Here's how the part is built. I have some questions about the finished solid (model axes, mm). A direction names the side the tool comes from. Round coordinates to 2 decimals unless told otherwise and drop trailing zeros. Order: outer loops, then holes, each group sorted by start corner. A loop starts at its lowest first (then second) coordinate and runs counter-clockwise, first axis right, second up.
```python
from build123d import *

# Parameters (mm, degrees)
BOSS_EXTRUDE1_DEPTH     = 3
BOSS_EXTRUDE2_DEPTH     = 132
CUT_EXTRUDE1_DEPTH      = 219.5
CUT_EXTRUDE1_DEPTH_BACK = 24.5
SKETCH3_W               = 129
SKETCH3_H               = 210
CUT_EXTRUDE2_DEPTH      = 322
CUT_EXTRUDE2_DEPTH_BACK = 22
SKETCH5_W               = 145
SKETCH5_H               = 129
BOSS_EXTRUDE3_DEPTH     = 10
BOSS_EXTRUDE4_DEPTH     = 15
CHAMFER1_SIZE           = 5
CHAMFER2_SIZE           = 3
CUT_EXTRUDE3_DEPTH      = 295
CUT_EXTRUDE3_DEPTH_BACK = 5
SKETCH10_R              = 2.5
SKETCH11_R              = 12
SKETCH11_R_2            = 7.6
SKETCH11_R_3            = 25
SKETCH11_R_4            = 1.6
CUT_EXTRUDE4_DEPTH      = 10
SKETCH13_R              = 4
CUT_EXTRUDE6_DEPTH      = 10


with BuildPart() as part:
    # Sketch1 → Boss-Extrude1 (new body)
    with BuildSketch(Plane.XY):
        with BuildLine():
            Line((15, 0), (235, 0))
            ThreePointArc((235, 0), (245.606601718, 4.393398282), (250, 15))
            Line((250, 15), (250, 335))
            ThreePointArc((250, 335), (245.606601718, 345.606601718), (235, 350))
            Line((235, 350), (15, 350))
            ThreePointArc((15, 350), (4.393398282, 345.606601718), (0, 335))
            Line((0, 335), (0, 15))
            ThreePointArc((0, 15), (4.393398282, 4.393398282), (15, 0))
        make_face()
    extrude(amount=BOSS_EXTRUDE1_DEPTH)

    # Sketch2 → Boss-Extrude2 (add)
    with BuildSketch(Plane.XY.offset(3)):
        with BuildLine():
            Line((0, 335), (0, 15))
            ThreePointArc((0, 15), (4.393398282, 4.393398282), (15, 0))
            Line((15, 0), (235, 0))
            ThreePointArc((235, 0), (245.606601718, 4.393398282), (250, 15))
            Line((250, 15), (250, 335))
            ThreePointArc((250, 335), (245.606601718, 345.606601718), (235, 350))
            Line((235, 350), (15, 350))
            ThreePointArc((15, 350), (4.393398282, 345.606601718), (0, 335))
        make_face()
        with BuildLine():
            ThreePointArc((32.5, 325), (28.964466094, 323.535533906), (27.5, 320))
            Line((27.5, 320), (27.5, 30))
            ThreePointArc((27.5, 30), (28.964466094, 26.464466094), (32.5, 25))
            Line((32.5, 25), (217.5, 25))
            ThreePointArc((217.5, 25), (221.035533906, 26.464466094), (222.5, 30))
            Line((222.5, 30), (222.5, 320))
            ThreePointArc((222.5, 320), (221.035533906, 323.535533906), (217.5, 325))
            Line((217.5, 325), (32.5, 325))
        make_face(mode=Mode.SUBTRACT)
    extrude(amount=BOSS_EXTRUDE2_DEPTH)

    # Sketch3 → Cut-Extrude1 (cut, two sides: drawn at the far end of the back side and taken through both)
    with BuildSketch(Plane(origin=(27.5, 0, 0), x_dir=(0, 0, -1), z_dir=(1, 0, 0)).offset(-CUT_EXTRUDE1_DEPTH_BACK)):
        with Locations((-67.5, 175)):
            Rectangle(SKETCH3_W, SKETCH3_H)
    extrude(amount=CUT_EXTRUDE1_DEPTH + CUT_EXTRUDE1_DEPTH_BACK, mode=Mode.SUBTRACT)

    # Sketch5 → Cut-Extrude2 (cut, two sides: drawn at the far end of the back side and taken through both)
    with BuildSketch(Plane(origin=(0, 25, 0), x_dir=(1, 0, 0), z_dir=(0, 1, 0)).offset(-CUT_EXTRUDE2_DEPTH_BACK)):
        with Locations((125, -67.5)):
            Rectangle(SKETCH5_W, SKETCH5_H)
    extrude(amount=CUT_EXTRUDE2_DEPTH + CUT_EXTRUDE2_DEPTH_BACK, mode=Mode.SUBTRACT)

    # Sketch8 → Boss-Extrude3 (add)
    with BuildSketch(Plane.XY.offset(135)):
        with BuildLine():
            Line((225.5, 30), (225.5, 320))
            ThreePointArc((225.5, 320), (223.156854249, 325.656854249), (217.5, 328))
            Line((217.5, 328), (32.5, 328))
            ThreePointArc((32.5, 328), (26.843145751, 325.656854249), (24.5, 320))
            Line((24.5, 320), (24.5, 30))
            ThreePointArc((24.5, 30), (26.843145751, 24.343145751), (32.5, 22))
            Line((32.5, 22), (217.5, 22))
            ThreePointArc((217.5, 22), (223.156854249, 24.343145751), (225.5, 30))
        make_face()
        with BuildLine():
            Line((32.5, 25), (217.5, 25))
            ThreePointArc((217.5, 25), (221.035533906, 26.464466094), (222.5, 30))
            Line((222.5, 30), (222.5, 320))
            ThreePointArc((222.5, 320), (221.035533906, 323.535533906), (217.5, 325))
            Line((217.5, 325), (32.5, 325))
            ThreePointArc((32.5, 325), (28.964466094, 323.535533906), (27.5, 320))
            Line((27.5, 320), (27.5, 30))
            ThreePointArc((27.5, 30), (28.964466094, 26.464466094), (32.5, 25))
        make_face(mode=Mode.SUBTRACT)
    extrude(amount=BOSS_EXTRUDE3_DEPTH)

    # Sketch9 → Boss-Extrude4 (add)
    with BuildSketch(Plane.XY.offset(135)):
        with BuildLine():
            ThreePointArc((0, 15), (4.393398282, 4.393398282), (15, 0))
            Line((15, 0), (30, 0))
            Line((30, 0), (30, 15))
            Line((30, 15), (15, 30))
            Line((15, 30), (0, 30))
            Line((0, 30), (0, 15))
        make_face()
        with BuildLine():
            Line((0, 335), (0, 320))
            Line((0, 320), (15, 320))
            Line((15, 320), (30, 335))
            Line((30, 335), (30, 350))
            Line((30, 350), (15, 350))
            ThreePointArc((15, 350), (4.393398282, 345.606601718), (0, 335))
        make_face()
    extrude(amount=BOSS_EXTRUDE4_DEPTH)

    # Chamfer1
    chamfer1_edges = [part.edges().sort_by_distance(p)[0] for p in [
        (0, 22.5, 150),
        (4.393398282, 4.393398282, 150),
        (22.5, 0, 150),
        (22.5, 350, 150),
        (4.393398282, 345.606601718, 150),
        (0, 327.5, 150),
    ]]
    chamfer(chamfer1_edges, length=CHAMFER1_SIZE)

    # Chamfer2
    chamfer2_edges = [part.edges().sort_by_distance(p)[0] for p in [
        (30, 10, 150),
        (22.5, 22.5, 150),
        (22.5, 327.5, 150),
        (30, 340, 150),
        (10, 30, 150),
        (10, 320, 150),
    ]]
    chamfer(chamfer2_edges, length=CHAMFER2_SIZE)

    # Sketch10 → Cut-Extrude3 (cut, two sides: drawn at the far end of the back side and taken through both)
    with BuildSketch(Plane(origin=(0, 30, 0), x_dir=(1, 0, 0), z_dir=(0, 1, 0)).offset(-CUT_EXTRUDE3_DEPTH_BACK)):
        with Locations(Location((7, -144, 0), (0, 0, 270))):
            Circle(SKETCH10_R)
    extrude(amount=CUT_EXTRUDE3_DEPTH + CUT_EXTRUDE3_DEPTH_BACK, mode=Mode.SUBTRACT)

    # Sketch11 → Cut-Extrude4 (cut)
    with BuildSketch(Plane(origin=(0, 3, 0), x_dir=(1, 0, 0), z_dir=(0, 1, 0))):
        with Locations(Location((160, -87.5, 0), (0, 0, 270))):
            Circle(SKETCH11_R)
        with Locations(Location((145, -47.5, 0), (0, 0, 270))):
            Circle(SKETCH11_R_2)
        with Locations(Location((175, -47.5, 0), (0, 0, 270))):
            Circle(SKETCH11_R_2)
        with Locations(Location((90, -67.5, 0), (0, 0, 270))):
            Circle(SKETCH11_R_3)
        with Locations(Location((150.5, -99.5, 0), (0, 0, 270))):
            Circle(SKETCH11_R_4)
        with Locations(Location((169.5, -75.5, 0), (0, 0, 270))):
            Circle(SKETCH11_R_4)
    extrude(amount=-CUT_EXTRUDE4_DEPTH, mode=Mode.SUBTRACT)

    # Sketch13 → Cut-Extrude6 (cut)
    with BuildSketch(Plane.ZY.offset(-247)):
        with Locations((67.5, 140)):
            Circle(SKETCH13_R)
        with BuildLine():
            Line((57.460079682, 173.9), (56.5, 173.9))
            Line((56.5, 173.9), (56.5, 176.1))
            Line((56.5, 176.1), (57.460079682, 176.1))
            ThreePointArc((57.460079682, 176.1), (77.6, 175), (57.460079682, 173.9))
        make_face()
    extrude(amount=-CUT_EXTRUDE6_DEPTH, mode=Mode.SUBTRACT)


solid = part.part
```
1. On a 3-axis mill with a long thin cutter (end or side, diameter ignored), from which of +Z, -Z, +X, -X, +Y, -Y can I reach the whole of each face in a straight line? I mean faces 1 (the cylindrical face through (248.48, 175.43, 77.59)), 2 (the flat face through (15, 174, 132)), 3 (the flat face through (234, 177, 135)), 4 (the flat face through (21.56, 21.35, 148.48)). Say none if no direction works.
Evaluation:
face 1: +X
face 2: none
face 3: +Z
face 4: +Z, +X
2. If we mould it in two halves opening along Y, with no side actions, what happens to faces 5 (the flat face through (197.5, 14, 68)), 6 (the flat face through (30, 7, 141)), 7 (the cylindrical face through (248.479, 143.373, 69.65)), 8 (the cylindrical face through (4.28, 4.51, 71.48))? For each: released by +Y, released by -Y, zero draft, split by the parting line, or undercut.
Evaluation:
face 5: undercut
face 6: zero draft
face 7: undercut
face 8: released by -Y
3. I'm going to push flat-ended pins straight in: P1, Ø3, axis at y = 120, z = 142.5, coming from the -X side; P2, Ø9.5, axis at y = 340.5, z = 143.5, coming from the +X side; P3, Ø10, axis at x = 98, y = 95.5, coming from the +Z side. Where does each tip first touch, or does it pass through?
Evaluation:
P1: stops at x = 24.5
P2: stops at x = 30
P3: stops at z = 3
4. If we section it at A-A, the plane x = 110: Write out the boundary of the cut face in (y, z).
Evaluation:
outline: (0, 0) - (350, 0) - (350, 135) - (328, 135) - (328, 145) - (325, 145) - (325, 132) - (347, 132) - (347, 3) - (3, 3) - (3, 52.5) - (0, 52.5) - close; (0, 82.5) - (3, 82.5) - (3, 132) - (25, 132) - (25, 145) - (22, 145) - (22, 135) - (0, 135) - close
5. If we section it at C-C, the plane y = 295: Write out the boundary of the cut face in (x, z), and give its area (3 significant figures).
Evaluation:
outline: (0, 0) - (250, 0) - (250, 135) - (225.5, 135) - (225.5, 145) - (222.5, 145) - (222.5, 3) - (27.5, 3) - (27.5, 145) - (24.5, 145) - (24.5, 135) - (0, 135) - close
area: 8,070 mm2
6. I need wall thicknesses on probe 1 along Y at (x, z) = (40.5, 129.5); probe 2 along Y at (x, z) = (118.5, 141); probe 3 along X at (y, z) = (268, 72). Which ranges of each line are inside material? Lowest first, please.
Evaluation:
probe 1: y = 0 to 25, 325 to 350
probe 2: y = 22 to 25, 325 to 328
probe 3: x = 0 to 3, 247 to 250
7. If we section it at D-D, the plane z = 67.5: State how many separate pieces and enclosed holes the cut face has, and give its area (3 significant figures).
Evaluation:
separate pieces: 3
enclosed holes: 0
area: 11,900 mm2
